```python
from build123d import *

# Parameters (mm, degrees)
SKETCH_1_R          = 9
SKETCH_1_R_2        = 1.25
EXTRUDE_1_DEPTH     = 10.25
SKETCH_2_R          = 2
CUT_EXTRUDE_1_DEPTH = 45


with BuildPart() as part:
    # 草圖1 → 填料-伸長1 (new body, symmetric)
    with BuildSketch(Plane(origin=(0, 0, 0), x_dir=(0, 0, -1), z_dir=(1, 0, 0))):
        with BuildLine():
            Line((-44, 0), (-44, -48.547028554))
            ThreePointArc((-44, -48.547028554), (-43.070090031, -51.286454985), (-40.664685703, -52.893694772))
            Line((-40.664685703, -52.893694772), (-27.771382825, -56.348444866))
            ThreePointArc((-27.771382825, -56.348444866), (-25.335277119, -56.231430318), (-23.419956354, -54.721513175))
            Line((-23.419956354, -54.721513175), (0, -20))
            Line((0, -20), (0, 0))
            Line((0, 0), (-44, 0))
        make_face()
        with Locations((-26, -26)):
            Circle(SKETCH_1_R, mode=Mode.SUBTRACT)
        with Locations((-36.5, -5.25)):
            Circle(SKETCH_1_R_2, mode=Mode.SUBTRACT)
        with Locations((-7.5, -5.25)):
            Circle(SKETCH_1_R_2, mode=Mode.SUBTRACT)
    extrude(amount=EXTRUDE_1_DEPTH, both=True)

    # 草圖2 → 除料-伸長1 (cut, through all)
    with BuildSketch(Plane.XY.offset(44)):
        with Locations((0, -10.5)):
            Circle(SKETCH_2_R)
    extrude(amount=-CUT_EXTRUDE_1_DEPTH, mode=Mode.SUBTRACT)


solid = part.part
```
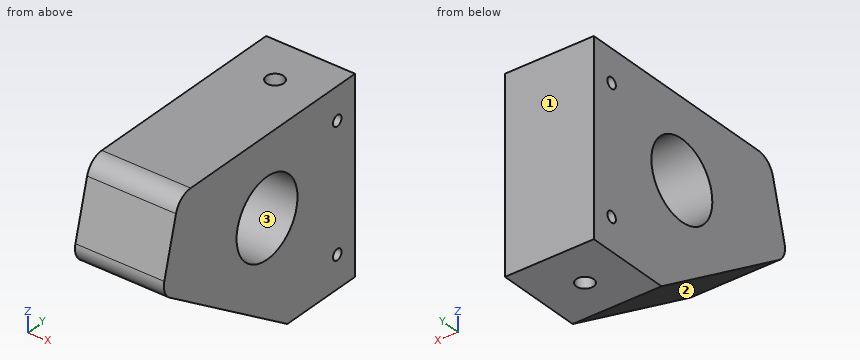
Read the model definition and answer for the solid it produces. Units are mm, in the model's axes. Face numbers are marked on the shaded views. Give positions to 0.01 mm unless a question says otherwise; leave off trailing zeros. Write each loop counter-clockwise with the first axis right and the second up, starting at its lowest first coordinate (ties: lowest second). Pieces come first, ordered by that corner, then holes. Notation, with made-up numbers: (28.25, 69) - (64.25, 69) arc R16 cw to (64.25, 80) - close; hole circle Ø1 at (-4.75, 16.5). An arc over 180 degrees is marked (long way). Write item = value, one per line. Start each with the question number.
Item 1: Find section A-A (x = 0). Give the vertices of the cut face in (y, z), then the cut area to 3 significant figures.
Item 2: Find section D-D (x = 3). Give the vertices of the cut face in (y, z), then the cut area to 3 significant figures.
Item 3: Find the intervals of material crossed by probe 1 along Z at (x, y) = (-0.25, -27); probe 2 along Z at (x, y) = (6.5, -20); probe 3 along Y at (x, z) = (0, 29.5), in increasing order. Write a range as [from, to].
Item 4: Each of these flat-tipped pins is pushed along its axis until it touches: P1, Ø2, axis at x = -5, y = -50, coming from the -Z side; P2, Ø4, axis at y = -5.25, z = 36.5, coming from the +X side; P3, Ø1.5, axis at y = -5.25, z = 7.5, coming from the +X side (3 decimals); P4, Ø5, axis at x = 4, z = 9.5, coming from the -Y side. Where does it stop, or does it pass through?
Item 5: Find section C-C (y = -10.5). Give the vertices of the cut face in (x, z).
Item 6: Find section B-B (z = 36.5). Give the vertices of the cut face in (x, y).
Item 7: The mould has two halves that part along Y. Classify the marked faces 1, 2 and 3: +Y half, -Y half, draft (parallel to the pull), parting line (faces both ways), or undercut.
Response:
q1.outline = (-56.35, 27.77) arc R4 ccw to (-54.72, 23.42) - (-20, 0) - (-12.5, 0) - (-12.5, 44) - (-48.55, 44) arc R4.5 ccw to (-52.89, 40.66) - close; (-8.5, 0) - (0, 0) - (0, 44) - (-8.5, 44) - close; hole circle Ø18 at (-26, 26); hole circle Ø2.5 at (-5.25, 7.5); hole circle Ø2.5 at (-5.25, 36.5)
q1.area = 1,560 mm²
q2.outline = (-56.35, 27.77) arc R4 ccw to (-54.72, 23.42) - (-20, 0) - (0, 0) - (0, 44) - (-48.55, 44) arc R4.5 ccw to (-52.89, 40.66) - close; hole circle Ø18 at (-26, 26); hole circle Ø2.5 at (-5.25, 7.5); hole circle Ø2.5 at (-5.25, 36.5)
q2.area = 1,730 mm²
q3.probe_1 = [4.72, 17.06], [34.94, 44]
q3.probe_2 = [0, 19.29], [32.71, 44]
q3.probe_3 = [-55.89, -34.29], [-17.71, -12.5], [-8.5, 0]
q4.P1 = 19.56
q4.P2 = 10.25
q4.P3 = through
q4.P4 = -37.79
q5.outline = (-10.25, 0) - (-2, 0) - (-2, 44) - (-10.25, 44) - close; (2, 0) - (10.25, 0) - (10.25, 44) - (2, 44) - close
q6.outline = (-10.25, -54.01) - (10.25, -54.01) - (10.25, -6.5) - (-10.25, -6.5) - close; (-10.25, -4) - (10.25, -4) - (10.25, 0) - (-10.25, 0) - close; hole circle Ø4 at (0, -10.5)
q7.face_1 = +Y half
q7.face_2 = -Y half
q7.face_3 = undercut
